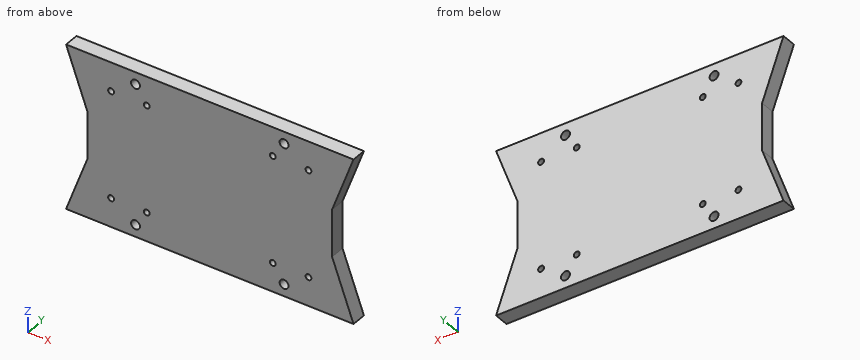
```python
from build123d import *

# Parameters (mm, degrees)
SKETCH10_R          = 1.905
BOSS_EXTRUDE2_DEPTH = 6.35
SKETCH11_R          = 1.2446
CUT_EXTRUDE1_DEPTH  = 6.35


with BuildPart() as part:
    # Sketch10 → Boss-Extrude2 (new body)
    with BuildSketch(Plane(origin=(0, 0, 0), x_dir=(1, 0, 0), z_dir=(0, 1, 0))):
        Polygon((0, 69.85), (9.144, 44.958), (9.144, 24.894999994), (0, 0), (61.443008686, 0), (61.443008686, 69.85), align=None)
        with Locations((29.693008686, 64.77)):
            Circle(SKETCH10_R, mode=Mode.SUBTRACT)
        with Locations((29.693008686, 5.08)):
            Circle(SKETCH10_R, mode=Mode.SUBTRACT)
    boss_extrude2 = extrude(amount=BOSS_EXTRUDE2_DEPTH)

    # Sketch11 → Cut-Extrude1 (cut)
    with BuildSketch(Plane(origin=(0, 6.35, 0), x_dir=(1, 0, 0), z_dir=(0, 1, 0))):
        with Locations((34.490278238, 57.62800006)):
            Circle(SKETCH11_R)
        with Locations((19.250278238, 57.62800006)):
            Circle(SKETCH11_R)
        with Locations((34.490278238, 12.224999934)):
            Circle(SKETCH11_R)
        with Locations((19.250278238, 12.224999934)):
            Circle(SKETCH11_R)
    cut_extrude1 = extrude(amount=-CUT_EXTRUDE1_DEPTH, mode=Mode.SUBTRACT)

    # Mirror3: Boss-Extrude2, Cut-Extrude1 across plane
    add(boss_extrude2.mirror(Plane(origin=(61.443008686, 6.35, 0), x_dir=(0, 0, 1), z_dir=(-1, 0, 0))))
    add(cut_extrude1.mirror(Plane(origin=(61.443008686, 6.35, 0), x_dir=(0, 0, 1), z_dir=(-1, 0, 0))), mode=Mode.SUBTRACT)


solid = part.part
```
Geometry check sheet. Reference: the model listing, model coordinates, mm. Round coordinates to 2 decimals unless told otherwise and drop trailing zeros. Loops run counter-clockwise (first coordinate to the right, second up) from the corner with the lowest first, then second, coordinate; pieces in that order, holes last. Notation, with made-up numbers: (68.5, 8.5) -> (112.5, 8.5) arc R15 cw to (112.5, 17.5) -> close; hole circle Ø3 at (-4, 52). An arc over 180 degrees is marked (long way). Use a Markdown table: item, result.
(1) Sectioned sample at B-B (y = 2.5). Give the number of separate pieces and of enclosed holes in the cut face, then the cut area to 3 significant figures.
Calculated:
| item | result |
|---|---|
| separate pieces | 1 |
| enclosed holes | 12 |
| area | 7,680 mm² |
(2) Go/stop test with flat-tipped pins: P1, Ø1.9, axis at y = 3.5, z = -33.5, coming from the -X side; P2, Ø1.5, axis at y = 2, z = -53.5, coming from the +X side. Record where each tip stops, or that it passes through.
Calculated:
| item | result |
|---|---|
| P1 | x = 9.14 |
| P2 | x = 117.16 |
(3) Sectioned sample at A-A (z = -5.08). Enter the section's corners in (x, y), then the cut area to 3 significant figures.
Calculated:
| item | result |
|---|---|
| outline | (1.87, 0) -> (27.79, 0) -> (27.79, 6.35) -> (1.87, 6.35) -> close; (31.6, 0) -> (91.29, 0) -> (91.29, 6.35) -> (31.6, 6.35) -> close; (95.1, 0) -> (121.02, 0) -> (121.02, 6.35) -> (95.1, 6.35) -> close |
| area | 708 mm² |
(4) Sectioned sample at D-D (z = -39.5). Enter the section's corners in (x, y), then the cut area to 3 significant figures.
Calculated:
| item | result |
|---|---|
| outline | (9.14, 0) -> (113.74, 0) -> (113.74, 6.35) -> (9.14, 6.35) -> close |
| area | 664 mm² |
(5) Scan lines: probe 1 along Z at (x, y) = (19, 5.5); probe 2 along X at (y, z) = (5.25, -57); probe 3 along Z at (x, y) = (30, 2). Record each from-to range of solid material in increasing order.
Calculated:
| item | result |
|---|---|
| probe 1 | -69.85 to -58.85, -56.41 to -13.44, -11.01 to 0 |
| probe 2 | 4.72 to 18.18, 20.32 to 33.42, 35.56 to 87.32, 89.47 to 102.56, 104.71 to 118.17 |
| probe 3 | -69.85 to -66.65, -62.89 to -6.96, -3.2 to 0 |
